Here's how the part is built. I have some questions about the finished solid (model axes, mm). A direction names the side the tool comes from. Coordinates: 2 decimals unless noted, no trailing zeros. Order: outer loops, then holes, each group sorted by start corner. A loop starts at its lowest first (then second) coordinate and runs counter-clockwise, first axis right, second up. Notation, with made-up numbers: (71, 4.5) -> (100, 4.5) arc R15 cw to (100, 32.5) -> close; hole circle Ø7 at (-11.5, -18.5). An arc over 180 degrees is marked (long way). One line per item, written item: value. Start each with the question number.
```python
from build123d import *

# Parameters (mm, degrees)
ESBO_O1_R                = 5.25
RESSALTO_EXTRUS_O1_DEPTH = 34.8
ESBO_O2_R                = 7.5
RESSALTO_EXTRUS_O2_DEPTH = 10
CORTE_EXTRUS_O1_DEPTH    = 5
ESBO_O4_R                = 5.25
CORTE_EXTRUS_O2_DEPTH    = 4


with BuildPart() as part:
    # Esboço1 → Ressalto-extrusão1 (new body)
    with BuildSketch(Plane(origin=(0, 0, 0), x_dir=(1, 0, 0), z_dir=(0, 1, 0))):
        Circle(ESBO_O1_R)
    extrude(amount=RESSALTO_EXTRUS_O1_DEPTH)

    # Esboço2 → Ressalto-extrusão2 (add)
    with BuildSketch(Plane(origin=(0, 34.8, 0), x_dir=(1, 0, 0), z_dir=(0, 1, 0))):
        Circle(ESBO_O2_R)
    extrude(amount=RESSALTO_EXTRUS_O2_DEPTH)

    # Esboço3 → Corte-extrusão1 (cut)
    with BuildSketch(Plane(origin=(0, 44.8, 0), x_dir=(1, 0, 0), z_dir=(0, 1, 0))):
        Polygon((0.212546418, 4.56974799), (-3.851244639, 2.468944592), (-4.063791057, -2.100803397), (-0.212546418, -4.56974799), (3.851244639, -2.468944592), (4.063791057, 2.100803397), align=None)
    extrude(amount=-CORTE_EXTRUS_O1_DEPTH, mode=Mode.SUBTRACT)

    # Esboço4 → Corte-extrusão2 (cut)
    with BuildSketch(Plane.XZ):
        Circle(ESBO_O4_R)
    extrude(amount=-CORTE_EXTRUS_O2_DEPTH, mode=Mode.SUBTRACT)


solid = part.part
```
Q1. Imagine slicing it at C-C (y = 7). Write out the boundary of the cut face in (x, z), plus the area to 3 significant figures.
Q2. If we mould it in two halves opening along Z, with no side actions, what happens to faces 4 (the face through (-1.791, 42.335, -3.534)), 5 (the face through (5, 19.2, -1.6)), 6 (the face through (3.2, 44.8, 3.2))? For each: +Z half, -Z half, draft (parallel to the pull), parting line (faces both ways), or undercut.
Q3. For P1, Ø1, axis at x = 2.5, y = 34.5, coming from the +Z side; P2, Ø6, axis at x = 3, y = 9.5, coming from the -Z side; P3, Ø2, axis at y = 31, z = -1.5, coming from the +X side, each with a flat end and sliding along its axis, tell me the tip position at first contact or that it passes through.
Q4. I need wall thicknesses on line 1 (Y direction, x = 7.25, z = -0.5); line 2 (Y direction, x = -1.25, z = 3.5); line 3 (Z direction, x = 0, y = 32.5). Which ranges of each line are inside material? Lowest first, please.
Q5. Imagine slicing it at A-A (z = 3.5). Write out the boundary of the cut face in (x, y).
Q6. For faces 1 (the face through (-7.493, 39.73, -0.33)), 2 (the face through (-3.956, 42.335, -0.216)), 3 (the face through (-1.8, 34.8, -5.1)), which set-ups out of +Z, -Z, +X, -X, +Y, -Y let a thin tool reach every point of the face, with its end or its side?
Q7. Imagine slicing it at D-D (x = 6.5). Write out the boundary of the cut face in (y, z).
Q8. Imagine slicing it at B-B (x = 1). Write out the boundary of the cut face in (y, z).
Completed:
1. outline: circle Ø10.5 at (0, 0)
1. area: 86.6 mm2
2. face 4: undercut
2. face 5: parting line
2. face 6: draft
3. P1: stops at z = 7.2
3. P2: stops at z = -5.25
3. P3: stops at x = 5.23
4. line 1: y = 34.8 to 44.8
4. line 2: y = 4 to 39.8
4. line 3: z = -5.25 to 5.25
5. outline: (-6.63, 34.8) -> (-3.91, 34.8) -> (-3.91, 4) -> (3.91, 4) -> (3.91, 34.8) -> (6.63, 34.8) -> (6.63, 44.8) -> (1.86, 44.8) -> (1.86, 39.8) -> (-1.88, 39.8) -> (-1.88, 44.8) -> (-6.63, 44.8) -> close
6. face 1: +Y, -Y
6. face 2: +Y
6. face 3: -Y
7. outline: (34.8, -3.74) -> (44.8, -3.74) -> (44.8, 3.74) -> (34.8, 3.74) -> close
8. outline: (4, -5.15) -> (34.8, -5.15) -> (34.8, -7.43) -> (44.8, -7.43) -> (44.8, -4.06) -> (39.8, -4.06) -> (39.8, 3.94) -> (44.8, 3.94) -> (44.8, 7.43) -> (34.8, 7.43) -> (34.8, 5.15) -> (4, 5.15) -> close
